CAD build for the part. Positions are in the model's coordinates, mm. Face numbers are marked on the shaded views. A direction names the side the tool comes from. Give positions to 0.01 mm unless a question says otherwise; leave off trailing zeros. Order: outer loops, then holes, each group sorted by start corner. A loop starts at its lowest first (then second) coordinate and runs counter-clockwise, first axis right, second up.
Item 1: Band-saw the part on D-D on x = 0.75. Give the cut face in (y, z), plus the area to 3 significant figures.
Item 2: Flat gauge pin, fed straight in: P1, Ø1.2, axis at x = -0.5, z = 1.5, coming from the +Y side. Where does the tip first touch, or does it go through?
Item 3: Band-saw the part on B-B on x = -4.25. Give the cut face in (y, z), plus the area to 3 significant figures.
Item 4: Wall check: L1, parallel to Y at x = 3, z = 2.7; L2, parallel to X at y = 0.25, z = 1.6; L3, parallel to X at y = 2.75, z = 0.95. Give the ranges that are in metal, low to high.
Item 5: Band-saw the part on A-A on y = 1.25. Give the cut face in (x, z), plus the area to 3 significant figures.
Item 6: Two-plate mould, pull along X, no slides. Class the marked faces 4, 5, 6 and 7: released by +X, released by -X, zero draft, split by the parting line, or undercut.
Item 7: Band-saw the part on C-C on z = 1.05. Give the cut face in (x, y).
Item 8: Which spindle directions (+Z, -Z, +X, -X, +Y, -Y) get a long thin tool onto all of the face, cutting with end or side? Do the marked faces 1, 2 and 3. Say none if no direction does.
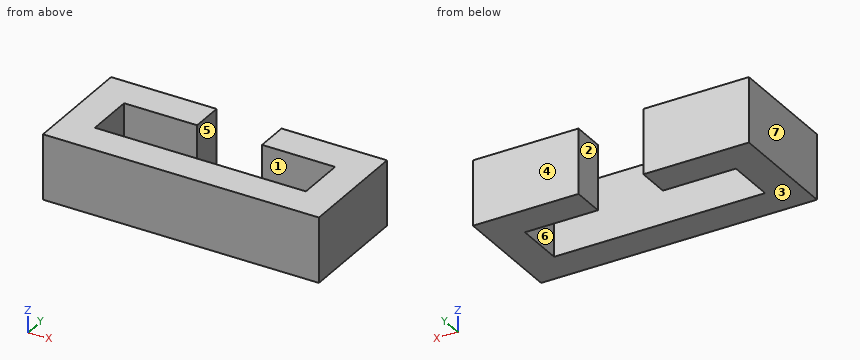
```python
from build123d import *

# Parameters (mm, degrees)
F0_W     = 17
F0_H     = 7
F0_W_2   = 13
F0_H_2   = 3
F1_DEPTH = 4
F2_W     = 4
F2_H     = 2
F3_DEPTH = 25


with BuildPart() as f1:
    # F0 (on Top) → F1 (new body)
    with BuildSketch(Plane.XY):
        Rectangle(F0_W, F0_H)
        Rectangle(F0_W_2, F0_H_2, mode=Mode.SUBTRACT)
    extrude(amount=F1_DEPTH)

    # F2 (on face) → F3 (cut)
    with BuildSketch(Plane.XY.offset(4)):
        with Locations((0, 2.5)):
            Rectangle(F2_W, F2_H)
    extrude(amount=-F3_DEPTH, mode=Mode.SUBTRACT)


solid = f1.part
```
The answers:
1. outline: (-3.5, 0) - (-1.5, 0) - (-1.5, 4) - (-3.5, 4) - close
1. area: 8.00 mm2
2. P1: stops at y = -1.5
3. outline: (-3.5, 0) - (-1.5, 0) - (-1.5, 4) - (-3.5, 4) - close; (1.5, 0) - (3.5, 0) - (3.5, 4) - (1.5, 4) - close
3. area: 16.0 mm2
4. L1: y = -3.5 to -1.5, 1.5 to 3.5
4. L2: x = -8.5 to -6.5, 6.5 to 8.5
4. L3: x = -8.5 to -2, 2 to 8.5
5. outline: (-8.5, 0) - (-6.5, 0) - (-6.5, 4) - (-8.5, 4) - close; (6.5, 0) - (8.5, 0) - (8.5, 4) - (6.5, 4) - close
5. area: 16.0 mm2
6. face 4: zero draft
6. face 5: undercut
6. face 6: undercut
6. face 7: released by -X
7. outline: (-8.5, -3.5) - (8.5, -3.5) - (8.5, 3.5) - (2, 3.5) - (2, 1.5) - (6.5, 1.5) - (6.5, -1.5) - (-6.5, -1.5) - (-6.5, 1.5) - (-2, 1.5) - (-2, 3.5) - (-8.5, 3.5) - close
8. face 1: +Z, -Z
8. face 2: +Z, -Z, +Y
8. face 3: -Z, +X, -X, +Y, -Y
